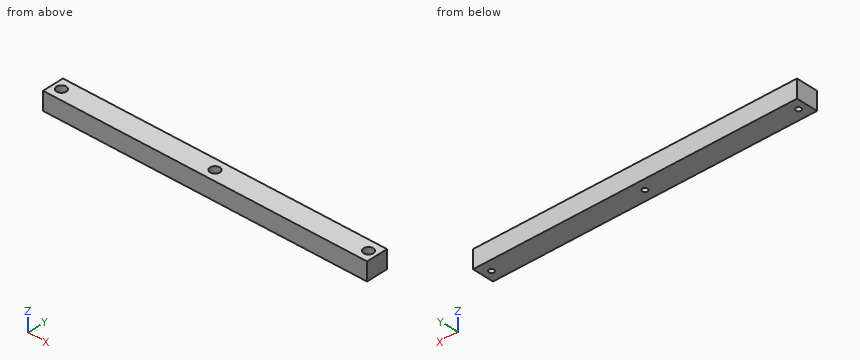
Autodesk Fusion 360 part; units mm, degrees
sketch "Sketch1" plane through (0, 0, 0) normal (0, 0, 1) x (1, 0, 0)
  line L0 (0, 0) -> (180, 0)
  line L1 (180, 0) -> (180, -12)
  line L2 (180, -12) -> (0, -12)
  line L3 (0, -12) -> (0, 0)
  dimension "d16" = 180
  dimension "d17" = 12
extrude "Extrude1" add sketch "Sketch1" along normal blind 10
sketch "Sketch6" plane through (0, 0, 10) normal (0, 0, 1) x (-1, 0, 0)
  line L0 (0, 12) -> (-180, 12)
  line L1 (-180, 12) -> (-180, 0)
  line L2 (-180, 0) -> (0, 0)
  line L3 (0, 0) -> (0, 12)
  circle A0 centre (-4.7, 6) radius 1.5
  circle A1 centre (-4.7, 6) radius 2.7
  circle A2 centre (-175.3, 6) radius 1.5
  circle A3 centre (-175.3, 6) radius 2.7
  line L4 (0, 12) -> (0, 0)
  line L5 (0, 0) -> (-180, 0)
  line L6 (-180, 0) -> (-180, 12)
  circle A4 centre (-90, 6) radius 1.5
  circle A5 centre (-90, 6) radius 2.7
  dimension "d65" = 3
  dimension "d66" = 1.2
  dimension "d67" = 3
  dimension "d68" = 1.2
  dimension "d69" = 4.7
  dimension "d70" = 6
  dimension "d71" = 4.7
  dimension "d72" = 6
  dimension "d82" = 3
  dimension "d83" = 1.2
  dimension "d88" = 6
  dimension "d89" = 90
extrude "Extrude9" cut sketch "Sketch6" against normal blind 100 contours A2
extrude "Extrude10" cut sketch "Sketch6" against normal blind 4 contours A3
extrude "Extrude11" cut sketch "Sketch6" against normal blind 100 contours A0
extrude "Extrude12" cut sketch "Sketch6" against normal blind 4 contours A1
extrude "Extrude13" cut sketch "Sketch6" against normal blind 100 contours A4
extrude "Extrude14" cut sketch "Sketch6" against normal blind 4 contours A5
equation "length = 180 mm"
equation "height = 10 mm"
equation "width = 12 mm"
equation "d16 = length"
equation "d17 = width"
equation "d18 = height"
equation "extra = 100 mm"
equation "bearing_outer_radius = 2.7 mm"
equation "bearing_width = 4 mm"
equation "bearing_big_distance = 2 mm + bearing_outer_radius"
equation "bearing_small_distance = width / 2"
equation "bearing_inner_radius = 1.5 mm"
equation "d65 = bearing_inner_radius * 2"
equation "d66 = bearing_outer_radius - bearing_inner_radius"
equation "d67 = bearing_inner_radius * 2"
equation "d68 = bearing_outer_radius - bearing_inner_radius"
equation "d69 = bearing_big_distance"
equation "d70 = bearing_small_distance"
equation "d71 = bearing_big_distance"
equation "d72 = bearing_small_distance"
equation "bearing_main_big_distance = length / 2"
equation "d82 = bearing_inner_radius * 2"
equation "d83 = bearing_outer_radius - bearing_inner_radius"
equation "d88 = bearing_small_distance"
equation "d89 = bearing_main_big_distance"
Build history of the part. All positions in model axes, mm. Coordinates: 2 decimals unless noted, no trailing zeros. Order: outer loops, then holes, each group sorted by start corner. A loop starts at its lowest first (then second) coordinate and runs counter-clockwise, first axis right, second up. Notation, with made-up numbers: (2.25, 71.25) - (8.25, 71.25) arc R22 ccw to (8.25, 108.25) - close; hole circle Ø8 at (-23.5, -38.75). An arc over 180 degrees is marked (long way). Write item = value, one per line. Start each with the question number.
1) Wall check: line 1 along X through (y, z) = (-6.25, 7); line 2 along Y through (x, z) = (175.3, 7); line 3 along Y through (x, z) = (90, 3.6). Give the ranges that are in metal, low to high. Write a range as from..to.
2) Saw through at B-B on y = -6. Write the cut outline in (x, z), then the cut area to 3 significant figures.
3) Flat gauge pin, fed straight in: pin 1 Ø5 at (x, y) = (175.3, -6) entering from +Z. Where does the tip first touch, or does it go through?
4) Saw through at A-A on x = 175.3. Write the cut outline in (y, z), then the cut area to 3 significant figures.
From the geometry:
q1.line_1 = 0..2.01, 7.39..87.31, 92.69..172.61, 177.99..180
q1.line_2 = -12..-8.7, -3.3..0
q1.line_3 = -12..-7.5, -4.5..0
q2.outline = (0, 0) - (3.2, 0) - (3.2, 6) - (2, 6) - (2, 10) - (0, 10) - close; (6.2, 0) - (88.5, 0) - (88.5, 6) - (87.3, 6) - (87.3, 10) - (7.4, 10) - (7.4, 6) - (6.2, 6) - close; (91.5, 0) - (173.8, 0) - (173.8, 6) - (172.6, 6) - (172.6, 10) - (92.7, 10) - (92.7, 6) - (91.5, 6) - close; (176.8, 0) - (180, 0) - (180, 10) - (178, 10) - (178, 6) - (176.8, 6) - close
q2.area = 1,680 mm^2
q3.pin_1 = 6
q4.outline = (-12, 0) - (-7.5, 0) - (-7.5, 6) - (-8.7, 6) - (-8.7, 10) - (-12, 10) - close; (-4.5, 0) - (0, 0) - (0, 10) - (-3.3, 10) - (-3.3, 6) - (-4.5, 6) - close
q4.area = 80.4 mm^2
